Geometry: final body of the model. Coordinates: model frame, mm. Face numbers are marked on the shaded views. A direction names the side the tool comes from. Give positions to 0.01 mm unless a question says otherwise; leave off trailing zeros. Loops run counter-clockwise (first coordinate to the right, second up) from the corner with the lowest first, then second, coordinate; pieces in that order, holes last. Notation, with made-up numbers: (-27.5, 87) - (31.5, 87) arc R18 ccw to (31.5, 104) - close; hole circle Ø4 at (75.5, 25.5). An arc over 180 degrees is marked (long way). Answer in a Markdown table with one row per item.
from build123d import *

# Parameters (mm, degrees)
SKETCH1_W           = 46.5
SKETCH1_H           = 34
BOSS_EXTRUDE1_DEPTH = 13.75
SKETCH2_W           = 46.5
SKETCH2_H           = 42.25
BOSS_EXTRUDE2_DEPTH = 2
CUT_EXTRUDE1_REACH  = 62.18
SKETCH3_R           = 1.25
SKETCH3_W           = 25
SKETCH3_H           = 10
SKETCH4_W           = 35
SKETCH4_H           = 12
CUT_EXTRUDE2_DEPTH  = 5
SKETCH6_R           = 2
CUT_EXTRUDE3_DEPTH  = 10
SKETCH7_W           = 25
SKETCH7_H           = 4
CUT_EXTRUDE4_DEPTH  = 10


with BuildPart() as part:
    # Sketch1 → Boss-Extrude1 (new body)
    with BuildSketch(Plane(origin=(0, 0, 0), x_dir=(1, 0, 0), z_dir=(0, 1, 0))):
        Rectangle(SKETCH1_W, SKETCH1_H)
    extrude(amount=BOSS_EXTRUDE1_DEPTH)

    # Sketch2 → Boss-Extrude2 (add)
    with BuildSketch(Plane.XY.offset(17)):
        with Locations((0, 21.125)):
            Rectangle(SKETCH2_W, SKETCH2_H)
    extrude(amount=BOSS_EXTRUDE2_DEPTH)

    # Sketch3 → Cut-Extrude1 (cut, up to next)
    with BuildSketch(Plane.XY.offset(19), mode=Mode.PRIVATE) as cut_extrude1_sk1:
        with Locations((-20, 39)):
            Circle(SKETCH3_R)
    cut_extrude1_tool1 = extrude(cut_extrude1_sk1.sketch, amount=-CUT_EXTRUDE1_REACH, mode=Mode.PRIVATE) & part.part
    # Sketch3 → Cut-Extrude1 (cut, up to next)
    with BuildSketch(Plane.XY.offset(19), mode=Mode.PRIVATE) as cut_extrude1_sk2:
        with Locations(Location((20, 39, 0), (0, 0, 180))):
            Circle(SKETCH3_R)
    cut_extrude1_tool2 = extrude(cut_extrude1_sk2.sketch, amount=-CUT_EXTRUDE1_REACH, mode=Mode.PRIVATE) & part.part
    # Sketch3 → Cut-Extrude1 (cut, up to next)
    with BuildSketch(Plane.XY.offset(19), mode=Mode.PRIVATE) as cut_extrude1_sk3:
        with Locations((20, 17)):
            Circle(SKETCH3_R)
    cut_extrude1_tool3 = extrude(cut_extrude1_sk3.sketch, amount=-CUT_EXTRUDE1_REACH, mode=Mode.PRIVATE) & part.part
    # Sketch3 → Cut-Extrude1 (cut, up to next)
    with BuildSketch(Plane.XY.offset(19), mode=Mode.PRIVATE) as cut_extrude1_sk4:
        with Locations(Location((-20, 17, 0), (0, 0, 180))):
            Circle(SKETCH3_R)
    cut_extrude1_tool4 = extrude(cut_extrude1_sk4.sketch, amount=-CUT_EXTRUDE1_REACH, mode=Mode.PRIVATE) & part.part
    # Sketch3 → Cut-Extrude1 (cut, up to next)
    with BuildSketch(Plane.XY.offset(19), mode=Mode.PRIVATE) as cut_extrude1_sk5:
        with Locations((0, 28)):
            Rectangle(SKETCH3_W, SKETCH3_H)
    cut_extrude1_tool5 = extrude(cut_extrude1_sk5.sketch, amount=-CUT_EXTRUDE1_REACH, mode=Mode.PRIVATE) & part.part
    add(cut_extrude1_tool1.solids().sort_by_distance((-20, 39, 19))[0], mode=Mode.SUBTRACT)
    add(cut_extrude1_tool2.solids().sort_by_distance((20, 39, 19))[0], mode=Mode.SUBTRACT)
    add(cut_extrude1_tool3.solids().sort_by_distance((20, 17, 19))[0], mode=Mode.SUBTRACT)
    add(cut_extrude1_tool4.solids().sort_by_distance((-20, 17, 19))[0], mode=Mode.SUBTRACT)
    add(cut_extrude1_tool5.solids().sort_by_distance((0, 28, 19))[0], mode=Mode.SUBTRACT)

    # Sketch4 → Cut-Extrude2 (cut)
    with BuildSketch(Plane(origin=(0, 13.75, 0), x_dir=(1, 0, 0), z_dir=(0, 1, 0))):
        with Locations((5.75, 0)):
            Rectangle(SKETCH4_W, SKETCH4_H)
    extrude(amount=-CUT_EXTRUDE2_DEPTH, mode=Mode.SUBTRACT)

    # Sketch6 → Cut-Extrude3 (cut)
    with BuildSketch(Plane.XZ):
        with Locations(Location((16.25, -10, 0), (0, 0, 270))):
            Circle(SKETCH6_R)
        with Locations(Location((16.25, 12, 0), (0, 0, 270))):
            Circle(SKETCH6_R)
        with Locations(Location((-16.25, -10, 0), (0, 0, 270))):
            Circle(SKETCH6_R)
        with Locations(Location((-16.25, 12, 0), (0, 0, 270))):
            Circle(SKETCH6_R)
    extrude(amount=-CUT_EXTRUDE3_DEPTH, mode=Mode.SUBTRACT)

    # Sketch7 → Cut-Extrude4 (cut)
    with BuildSketch(Plane(origin=(0, 0, 17), x_dir=(-1, 0, 0), z_dir=(0, 0, -1))):
        with Locations((0, 15.75)):
            Rectangle(SKETCH7_W, SKETCH7_H)
        with Locations((0, 40.25)):
            Rectangle(SKETCH7_W, SKETCH7_H)
    extrude(amount=-CUT_EXTRUDE4_DEPTH, mode=Mode.SUBTRACT)


solid = part.part
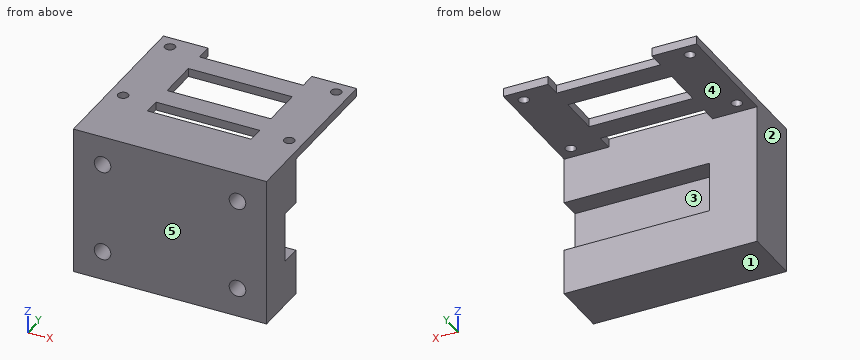
Q1. Material intervals for line 1 along X through (y, z) = (7.75, -10); line 2 along Y through (x, z) = (-20, 17.7); line 3 along Z through (x, y) = (16, 5), sorted ascending.
Check values:
| item | result |
|---|---|
| line 1 | -23.25 to -18.25, -14.25 to 14.25, 18.25 to 23.25 |
| line 2 | 0 to 15.75, 18.25 to 37.75, 40.25 to 42.25 |
| line 3 | -17 to -11.98, -8.02 to 10.02, 13.98 to 19 |
Q2. Cut plane A-A (y = 17). Output: boundary loops of the cut face in (x, z).
Check values:
| item | result |
|---|---|
| outline | (-23.25, 17) - (-21.25, 17) - (-21.25, 19) - (-23.25, 19) - close; (-18.75, 17) - (-12.5, 17) - (-12.5, 19) - (-18.75, 19) - close; (12.5, 17) - (18.75, 17) - (18.75, 19) - (12.5, 19) - close; (21.25, 17) - (23.25, 17) - (23.25, 19) - (21.25, 19) - close |
Q3. Reachability of the marked faces 4 and 5 from +Z, -Z, +X, -X, +Y, -Y: full face, straight path, thin tool, end or side. Return the list, or none.
Check values:
| item | result |
|---|---|
| face 4 | -Z, +X, -X, +Y |
| face 5 | +Z, -Z, +X, -X, -Y |
Q4. First-contact query: pin 1 (3 mm diameter, centred on x = -20, y = 17, fed in from +Z); pin 2 (1.2 mm diameter, centred on x = -17, z = -9, fed in from -Y); pin 3 (1.5 mm diameter, centred on x = 11, z = 7.5, fed in from +Y); pin 4 (6 mm diameter, centred on x = 10, z = 1.5, fed in from +Y). Flat tips, straight axial feed; report the tip coordinate or a pass-through.
Check values:
| item | result |
|---|---|
| pin 1 | z = 19 |
| pin 2 | y = 10 |
| pin 3 | y = 13.75 |
| pin 4 | y = 8.75 |
Q5. Cut plane B-B (x = 20). Output: boundary loops of the cut face in (y, z), and give its area (3 significant figures).
Check values:
| item | result |
|---|---|
| outline | (0, -17) - (13.75, -17) - (13.75, -6) - (8.75, -6) - (8.75, 6) - (13.75, 6) - (13.75, 17) - (15.75, 17) - (15.75, 19) - (0, 19) - close; (18.25, 17) - (37.75, 17) - (37.75, 19) - (18.25, 19) - close; (40.25, 17) - (42.25, 17) - (42.25, 19) - (40.25, 19) - close |
| area | 482 mm² |
Q6. Cut plane C-C (y = 4). Output: boundary loops of the cut face in (x, z).
Check values:
| item | result |
|---|---|
| outline | (-23.25, -17) - (23.25, -17) - (23.25, 19) - (-23.25, 19) - close; hole circle Ø4 at (-16.25, -10); hole circle Ø4 at (-16.25, 12); hole circle Ø4 at (16.25, -10); hole circle Ø4 at (16.25, 12) |
Q7. Cut plane D-D (x = -20). Output: boundary loops of the cut face in (y, z), and give its area (3 significant figures).
Check values:
| item | result |
|---|---|
| outline | (0, -17) - (13.75, -17) - (13.75, 17) - (15.75, 17) - (15.75, 19) - (0, 19) - close; (18.25, 17) - (37.75, 17) - (37.75, 19) - (18.25, 19) - close; (40.25, 17) - (42.25, 17) - (42.25, 19) - (40.25, 19) - close |
| area | 542 mm² |
Q8. Draft query along Z for the marked faces 1, 2 and 3. Return one class per face: pulls with the +Z half, pulls with the -Z half, needs draft (parallel to the pull), parting line crosses it, or undercut.
Check values:
| item | result |
|---|---|
| face 1 | pulls with the -Z half |
| face 2 | needs draft |
| face 3 | undercut |
